The listing builds one solid part. Answer for the finished solid, in the listing's coordinates (mm). Face numbers are marked on the shaded views. A direction names the side the tool comes from. Round coordinates to 2 decimals unless told otherwise and drop trailing zeros. Write each loop counter-clockwise with the first axis right and the second up, starting at its lowest first coordinate (ties: lowest second). Pieces come first, ordered by that corner, then holes. Notation, with made-up numbers: (-17.75, -36) - (40.25, -36) arc R17 cw to (40.25, -12) - close; hole circle Ø6 at (49, 64.25). An arc over 180 degrees is marked (long way). Return JSON: item names as keys, results as strings. Group by question number.
(1) Section A-A, the plane z = 0 is taken. Give the number of separate pieces and of enclosed holes in the cut face, then the cut area to 3 significant figures.
(2) Determine the mould class of the marked faces 1, 2 and 3 for opening direction Z: +Z half, -Z half, draft (parallel to the pull), parting line (faces both ways), or undercut.
(3) Section B-B, the plane x = 1 is taken. Write down the section's boundary in (y, z), then the cut area to 3 significant figures.
(4) Which of the six approach directions +Z, -Z, +X, -X, +Y, -Y give full straight-line access (tool end or side, diameter ignored) to the marked faces 4 and 5?
(5) Section C-C, the plane x = 18 is taken. Write down the section's boundary in (y, z).
(6) Each of these flat-tipped pins is pushed along its axis until it touches: pin 1 (3.5 mm diameter, centred on x = -25.5, z = -0.5, fed in from +Y); pin 2 (1.3 mm diameter, centred on x = 1, y = -3, fed in from +Z); pin 3 (1 mm diameter, centred on x = -16.5, y = -1.5, fed in from +Z). Where does it stop, or does it pass through?
(7) Find the intervals of material crossed by line 1 along X through (y, z) = (-3.85, 0) (3 decimals); line 2 along X through (y, z) = (-1.95, 0) (3 decimals); line 3 along Z through (x, y) = (26, -1.95), in increasing order. Write a range as [from, to].
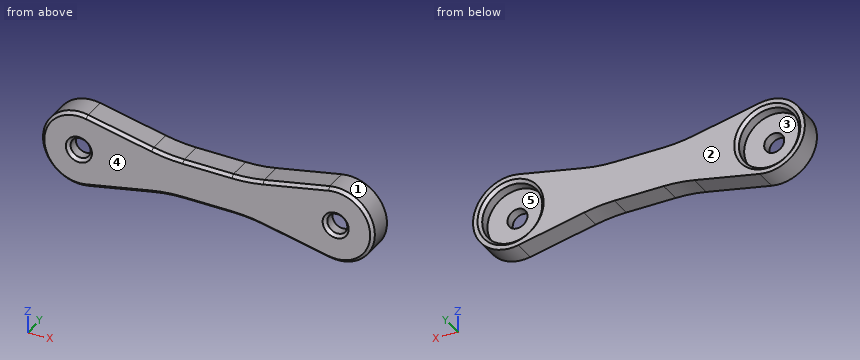
```python
from build123d import *

# Parameters (mm, degrees)
SKETCH1_R           = 2
BOSS_EXTRUDE1_DEPTH = 5
SKETCH1_3_R         = 6
CUT_EXTRUDE1_DEPTH  = 2.5
FILLET1_R           = 30
CHAMFER1_SIZE       = 0.6
CHAMFER2_SIZE       = 0.6


with BuildPart() as part:
    # Sketch1 → Boss-Extrude1 (new body)
    with BuildSketch(Plane(origin=(0, 0, 0), x_dir=(1, 0, 0), z_dir=(0, 1, 0))):
        with BuildLine():
            Line((-8, 4), (8, 4))
            Line((8, 4), (24.100084087, 7.343339258))
            ThreePointArc((24.100084087, 7.343339258), (33.125, 0), (24.100084087, -7.343339258))
            Line((24.100084087, -7.343339258), (8, -4))
            Line((8, -4), (-8, -4))
            Line((-8, -4), (-24.100084087, -7.343339258))
            ThreePointArc((-24.100084087, -7.343339258), (-33.125, 0), (-24.100084087, 7.343339258))
            Line((-24.100084087, 7.343339258), (-8, 4))
        make_face()
        with Locations(Location((-25.625, 0, 0), (0, 0, 270))):
            Circle(SKETCH1_R, mode=Mode.SUBTRACT)
        with Locations(Location((25.625, 0, 0), (0, 0, 270))):
            Circle(SKETCH1_R, mode=Mode.SUBTRACT)
    extrude(amount=-BOSS_EXTRUDE1_DEPTH)

    # Sketch1_3 → Cut-Extrude1 (cut)
    with BuildSketch(Plane(origin=(0, 0, 0), x_dir=(1, 0, 0), z_dir=(0, 1, 0))):
        with Locations(Location((25.625, 0, 0), (0, 0, 270))):
            Circle(SKETCH1_3_R)
        with Locations(Location((-25.625, 0, 0), (0, 0, 270))):
            Circle(SKETCH1_3_R)
    extrude(amount=-CUT_EXTRUDE1_DEPTH, mode=Mode.SUBTRACT)

    # Fillet1
    fillet1_edges = [part.edges().sort_by_distance(p)[0] for p in [
        (-8, -2.5, 4),
        (8, -2.5, 4),
        (8, -2.5, -4),
        (-8, -2.5, -4),
    ]]
    fillet(fillet1_edges, radius=FILLET1_R)

    # Chamfer1
    chamfer1_edges = [part.edges().sort_by_distance(p)[0] for p in [
        (17.558863569, -5, -5.984991113),
        (33.125, -5, 0),
        (17.558863569, -5, 5.984991113),
        (-25.625, -5, -2),
        (25.625, -5, -2),
        (-17.558863569, -5, 5.984991113),
        (-33.125, -5, 0),
        (0, -5, -4),
        (-17.558863569, -5, -5.984991113),
        (0, -5, 4),
        (7.983863369, -5, -4.157071935),
        (-7.983863369, -5, -4.157071935),
        (7.983863369, -5, 4.157071935),
        (-7.983863369, -5, 4.157071935),
    ]]
    chamfer(chamfer1_edges, length=CHAMFER1_SIZE)

    # Chamfer2
    chamfer2_edges = [part.edges().sort_by_distance(p)[0] for p in [
        (25.625, 0, -6),
        (-25.625, 0, -6),
    ]]
    chamfer(chamfer2_edges, length=CHAMFER2_SIZE)


solid = part.part
```
Working result:
{
 "1": {"separate pieces": "3", "enclosed holes": "0", "area": "249 mm^2"},
 "2": {"face 1": "parting line", "face 2": "draft", "face 3": "undercut"},
 "3": {"outline": "(-5, -3.4) - (-4.4, -4) - (0, -4) - (0, 4) - (-4.4, 4) - (-5, 3.4) - close", "area": "39.6 mm^2"},
 "4": {"face 4": "+Z, -Z, +X, -X, -Y", "face 5": "+Y"},
 "5": {"outline": "(-5, -5.46) - (-4.4, -6.08) - (0, -6.08) - (0, 6.08) - (-4.4, 6.08) - (-5, 5.46) - close"},
 "6": {"pin 1": "stops at y = -2.5", "pin 2": "stops at z = 4", "pin 3": "stops at z = 5.87"},
 "7": {"line 1": "x = [-33.125, -27.625], [-23.625, 23.625], [27.625, 33.125]", "line 2": "x = [-33.125, -31.625], [-19.625, 19.625], [31.625, 33.125]", "line 3": "z = [-7.49, -5.99], [5.99, 7.49]"}
}
